The figure shows three views and two pictorial views of one solid part (mm, origin at its lowest corner). Answer the questions. A direction names the side the tool comes from. Coordinates: 2 decimals unless noted, no trailing zeros. Loops run counter-clockwise (first coordinate to the right, second up) from the corner with the lowest first, then second, coordinate; pieces in that order, holes last. Notation, with made-up numbers: M -3,9.5 L 41,9.5 A34 ccw 41,44.5 Z; hole C 14.25,-34 d10. An arc over 180 degrees is marked long. One line per item, written item: value. Start each with the question number.
1. The part is cut by section B-B (z = 18). Write down the section's boundary in (x, y), then the cut area to 3 significant figures.
2. Consider probe 1 along X at (y, z) = (23.5, 31.5); probe 2 along Z at (x, y) = (45, 4) (1 decimal); probe 3 along X at (y, z) = (18, 46) (1 decimal). Determine where each line is inside the solid, lowest interval first.
3. Determine the mould class of the marked faces 3, 4 and 5 for opening direction X: +X half, -X half, draft (parallel to the pull), parting line (faces both ways), or undercut.
4. For the marked faces 1 and 2, determine the directions among +Z, -Z, +X, -X, +Y, -Y from which every point of the face is accessible in a straight line to the end or side of a thin tool.
5. The part is cut by section C-C (y = 35.5). Write down the section's boundary in (x, z), then the cut area to 3 significant figures.
6. The part is cut by section D-D (x = 54.5). Write down the section's boundary in (y, z), then the cut area to 3 significant figures.
7. The part is cut by section A-A (x = 19.5). Write down the section's boundary in (y, z), then the cut area to 3 significant figures.
8. Flat-ended cylindrical pins translate along their axes: pin 1 (5 mm diameter, centred on y = 8, z = 27, fed in from +X); pin 2 (3 mm diameter, centred on y = 8.5, z = 7, fed in from +X) (1 decimal); pin 3 (2 mm diameter, centred on y = 34.5, z = 19, fed in from -X) (1 decimal). Find the tip coordinate at first contact, or state that the pin passes through.
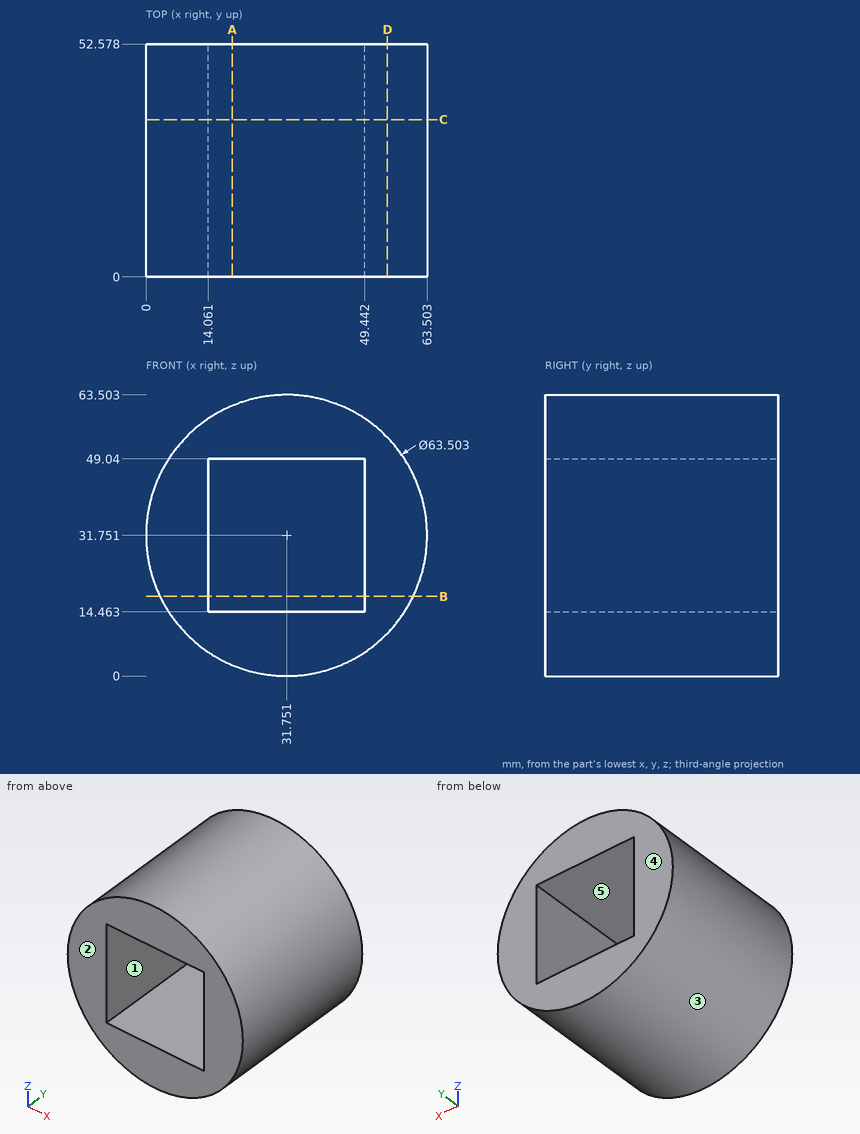
Answer block:
1. outline: M 3.13,0 L 14.06,0 L 14.06,52.58 L 3.13,52.58 Z; M 49.44,0 L 60.37,0 L 60.37,52.58 L 49.44,52.58 Z
1. area: 1,150 mm2
2. probe 1: x = 0 to 14.06, 49.44 to 63.5
2. probe 2: z = 2.9 to 14.5, 49 to 60.6
2. probe 3: x = 3.4 to 14.1, 49.4 to 60.1
3. face 3: parting line
3. face 4: draft
3. face 5: undercut
4. face 1: +Y, -Y
4. face 2: +Z, -Z, +X, -X, -Y
5. outline: C 31.75,31.75 d63.5; hole M 14.06,14.46 L 49.44,14.46 L 49.44,49.04 L 14.06,49.04 Z
5. area: 1,940 mm2
6. outline: M 0,9.6 L 52.58,9.6 L 52.58,53.9 L 0,53.9 Z
6. area: 2,330 mm2
7. outline: M 0,2.46 L 52.58,2.46 L 52.58,14.46 L 0,14.46 Z; M 0,49.04 L 52.58,49.04 L 52.58,61.04 L 0,61.04 Z
7. area: 1,260 mm2
8. pin 1: stops at x = 63.42
8. pin 2: stops at x = 53.4
8. pin 3: stops at x = 2.3
